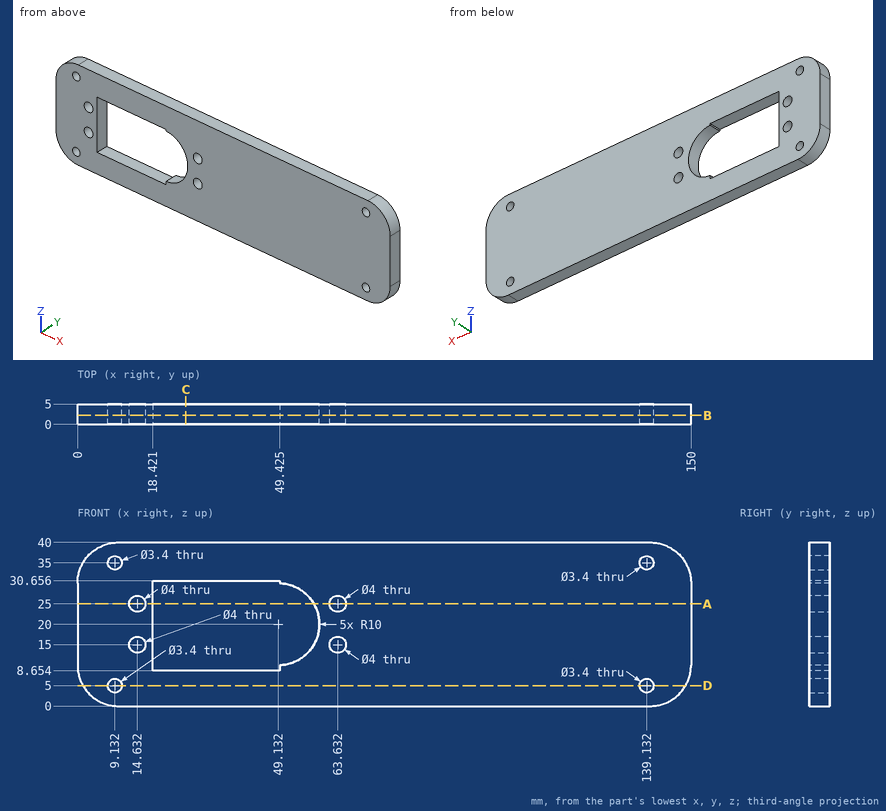
Answer from the drawing. Dimensions are ordinates in mm from the lowest x, y and z of the part. Coordinates: 2 decimals unless noted, no trailing zeros. Order: outer loops, then holes, each group sorted by start corner. A loop starts at its lowest first (then second) coordinate and runs counter-clockwise, first axis right, second up. Notation, with made-up numbers: (-6.75, 69.25) - (16.25, 69.25) arc R21 cw to (16.25, 107.25) - close; hole circle Ø1 at (2, 37.5). An arc over 180 degrees is marked (long way). Answer as a JSON object with one key per item and string values. Group by question number.
Item 1: Section D-D (z = 5) is taken. Give the vertices of the cut face in (x, y).
Item 2: Section B-B (y = 2.2) is taken. State how many separate pieces and enclosed holes the cut face has, plus the area to 3 significant figures.
Item 3: Section A-A (z = 25) is taken. Give the vertices of the cut face in (x, y).
Item 4: Section C-C (x = 26.5) is taken. Give the vertices of the cut face in (y, z), plus the area to 3 significant figures.
Item 5: Consider probe 1 along Z at (x, y) = (34.5, 3.7); probe 2 along Z at (x, y) = (10, 0.4); probe 3 along Z at (x, y) = (139, 3.8) (1 decimal). Determine where each line is inside the solid, lowest interval first. Write a range as from..to.
Results are:
{
 "1": {"outline": "(1.34, 0) - (7.43, 0) - (7.43, 5) - (1.34, 5) - close; (10.83, 0) - (137.43, 0) - (137.43, 5) - (10.83, 5) - close; (140.83, 0) - (148.66, 0) - (148.66, 5) - (140.83, 5) - close"},
 "2": {"separate pieces": "1", "enclosed holes": "9", "area": "4,990 mm^2"},
 "3": {"outline": "(0, 0) - (12.63, 0) - (12.63, 5) - (0, 5) - close; (16.63, 0) - (18.42, 0) - (18.42, 5) - (16.63, 5) - close; (57.79, 0) - (61.63, 0) - (61.63, 5) - (57.79, 5) - close; (65.63, 0) - (150, 0) - (150, 5) - (65.63, 5) - close"},
 "4": {"outline": "(0, 0) - (5, 0) - (5, 8.66) - (0, 8.66) - close; (0, 30.66) - (5, 30.66) - (5, 40) - (0, 40) - close", "area": "90.0 mm^2"},
 "5": {"probe 1": "z = 0..8.66, 30.66..40", "probe 2": "z = 0..3.54, 6.46..33.54, 36.46..40", "probe 3": "z = 0..3.3, 6.7..33.3, 36.7..40"}
}
